Part model, mm, in its own coordinate system. A direction names the side the tool comes from. Give positions to 0.01 mm unless a question says otherwise; leave off trailing zeros. Loops run counter-clockwise (first coordinate to the right, second up) from the corner with the lowest first, then second, coordinate; pieces in that order, holes last. Notation, with made-up numbers: M 59,32 L 103,32 A24 ccw 103,58 Z; hole C 14.25,58 d6. An arc over 180 degrees is marked long. Answer in a Markdown table with one row per item.
from build123d import *

# Parameters (mm, degrees)
BOSS_EXTRUDE1_DEPTH     = 12
SKETCH5_R               = 1
CUT_EXTRUDE1_DEPTH      = 10
CUT_EXTRUDE2_DEPTH      = 3
CUT_EXTRUDE2_DEPTH_BACK = 3
CUT_EXTRUDE3_DEPTH      = 21.976176963
CUT_EXTRUDE3_DEPTH_BACK = 21.976176963
SKETCH7_R               = 1.5
SKETCH10_W              = 7
SKETCH10_H              = 3
CUT_EXTRUDE4_DEPTH      = 3
SKETCH9_R               = 1
CUT_EXTRUDE5_DEPTH      = 27.981475126
SKETCH12_R              = 3
CUT_EXTRUDE6_DEPTH      = 6.5
CUT_EXTRUDE7_DEPTH      = 6.5


with BuildPart() as part:
    # Sketch2 → Boss-Extrude1 (new body)
    with BuildSketch(Plane(origin=(0, 0, 0), x_dir=(1, 0, 0), z_dir=(0, 1, 0))):
        Polygon((0, 10), (11, 10), (11, 0), (-11, 0), (-11, 10), align=None)
    extrude(amount=BOSS_EXTRUDE1_DEPTH)

    # Sketch5 → Cut-Extrude1 (cut)
    with BuildSketch(Plane(origin=(0, 0, -10), x_dir=(-1, 0, 0), z_dir=(0, 0, -1))):
        with Locations((9.5, 1.5)):
            Circle(SKETCH5_R)
    cut_extrude1 = extrude(amount=-CUT_EXTRUDE1_DEPTH, mode=Mode.SUBTRACT)

    # Sketch6 → Cut-Extrude2 (cut, two sides: drawn at the far end of the back side and taken through both)
    with BuildSketch(Plane(origin=(0, 0, 0), x_dir=(0, 0, -1), z_dir=(1, 0, 0)).offset(-CUT_EXTRUDE2_DEPTH_BACK)):
        with BuildLine():
            Line((6, 9.2), (10, 9.2))
            Line((10, 9.2), (10, 2.8))
            Line((10, 2.8), (6, 2.8))
            ThreePointArc((6, 2.8), (2.8, 6), (6, 9.2))
        make_face()
    extrude(amount=CUT_EXTRUDE2_DEPTH + CUT_EXTRUDE2_DEPTH_BACK, mode=Mode.SUBTRACT)

    # Sketch7 → Cut-Extrude3 (cut, two sides: drawn at the far end of the back side and taken through both)
    with BuildSketch(Plane.ZY.offset(-3).offset(-CUT_EXTRUDE3_DEPTH_BACK)):
        with Locations((-6, 6)):
            Circle(SKETCH7_R)
    extrude(amount=CUT_EXTRUDE3_DEPTH + CUT_EXTRUDE3_DEPTH_BACK, mode=Mode.SUBTRACT)

    # Sketch10 → Cut-Extrude4 (cut)
    with BuildSketch(Plane(origin=(0, 0, 0), x_dir=(1, 0, 0), z_dir=(0, 1, 0))):
        with Locations((-7.5, 1.5)):
            Rectangle(SKETCH10_W, SKETCH10_H)
    cut_extrude4 = extrude(amount=CUT_EXTRUDE4_DEPTH, mode=Mode.SUBTRACT)

    # Sketch9 → Cut-Extrude5 (cut, through all)
    with BuildSketch(Plane.ZY.offset(11)):
        with Locations((-1.5, 1.5)):
            Circle(SKETCH9_R)
    extrude(amount=-CUT_EXTRUDE5_DEPTH, mode=Mode.SUBTRACT)

    # Mirror1: Cut-Extrude1, Cut-Extrude4 across plane
    add(cut_extrude1.mirror(Plane(origin=(0, 0, 0), x_dir=(0, 0, 1), z_dir=(1, 0, 0))), mode=Mode.SUBTRACT)
    add(cut_extrude4.mirror(Plane(origin=(0, 0, 0), x_dir=(0, 0, 1), z_dir=(1, 0, 0))), mode=Mode.SUBTRACT)

    # Sketch12 → Cut-Extrude6 (cut)
    with BuildSketch(Plane(origin=(11, 0, 0), x_dir=(0, 0, -1), z_dir=(1, 0, 0))):
        with Locations((6, 6)):
            Circle(SKETCH12_R)
    extrude(amount=-CUT_EXTRUDE6_DEPTH, mode=Mode.SUBTRACT)

    # Sketch13 → Cut-Extrude7 (cut)
    with BuildSketch(Plane.ZY.offset(11)):
        Polygon((-9, 7.732050808), (-9, 4.267949192), (-6, 2.535898385), (-3, 4.267949192), (-3, 7.732050808), (-6, 9.464101615), align=None)
    extrude(amount=-CUT_EXTRUDE7_DEPTH, mode=Mode.SUBTRACT)


solid = part.part
(1) Which spindle directions (+Z, -Z, +X, -X, +Y, -Y) get a long thin tool onto all of the face, cutting with end or side? Do faces 1 (the face through (-7.8, 3.4, -4.5)), 2 (the face through (-8, 3, -2)), 3 (the face through (8, 1, -3)). Say none if no direction does.
Recorded:
| item | result |
|---|---|
| face 1 | -X |
| face 2 | +Z, -X, -Y |
| face 3 | +Z, +X, -Y |
(2) Saw through at C-C (z = -1.5). Write the cut outline in (x, y).
Recorded:
| item | result |
|---|---|
| outline | M -11,3 L -4,3 L -4,2.5 L 4,2.5 L 4,3 L 11,3 L 11,12 L -11,12 Z; M -4,0 L 4,0 L 4,0.5 L -4,0.5 Z |
(3) Saw through at D-D (x = 9.5). Write the cut outline in (y, z).
Recorded:
| item | result |
|---|---|
| outline | M 0,-10 L 0.5,-10 L 0.5,-3 L 0,-3 Z; M 2.5,-10 L 12,-10 L 12,0 L 3,0 L 3,-3 L 2.5,-3 Z; hole C 6,-6 d6 |
(4) Saw through at B-B (y = 1.5). Write the cut outline in (x, z), plus the area to 3 significant figures.
Recorded:
| item | result |
|---|---|
| outline | M -11,-10 L -10.5,-10 L -10.5,-3 L -11,-3 Z; M -8.5,-10 L 8.5,-10 L 8.5,-3 L 4,-3 L 4,-2.5 L -4,-2.5 L -4,-3 L -8.5,-3 Z; M -4,-0.5 L 4,-0.5 L 4,0 L -4,0 Z; M 10.5,-10 L 11,-10 L 11,-3 L 10.5,-3 Z |
| area | 134 mm^2 |
(5) Pull direction X, two halves, no side cores. Call faces 4 (the face through (7.796, 3.338, -7.384)), 5 (the face through (-11, 5.9, -2.7)), 6 (the face through (-8.7, 0.9, -6.5)): +X half, -X half, draft (parallel to the pull), parting line (faces both ways), or undercut.
Recorded:
| item | result |
|---|---|
| face 4 | draft |
| face 5 | -X half |
| face 6 | undercut |
(6) Pin check, flat tips, straight feed: pin 1 Ø0.9 at (x, y) = (8, 1) entering from +Z; pin 2 Ø1.6 at (y, z) = (1.5, -1.5) entering from -X; pin 3 Ø1.5 at (x, z) = (-6, -2) entering from -Y; pin 4 Ø3 at (y, z) = (4.5, -6) entering from -X. Stop position of each tip, or through.
Recorded:
| item | result |
|---|---|
| pin 1 | stops at z = -3 |
| pin 2 | passes through |
| pin 3 | stops at y = 3 |
| pin 4 | stops at x = -4.5 |
(7) Saw through at A-A (x = -9.5). Write the cut outline in (y, z), plus the area to 3 significant figures.
Recorded:
| item | result |
|---|---|
| outline | M 0,-10 L 0.5,-10 L 0.5,-3 L 0,-3 Z; M 2.5,-10 L 12,-10 L 12,0 L 3,0 L 3,-3 L 2.5,-3 Z; hole M 2.54,-6 L 4.27,-9 L 7.73,-9 L 9.46,-6 L 7.73,-3 L 4.27,-3 Z |
| area | 65.8 mm^2 |
(8) Drill centre lines: line 1 along Z through (x, y) = (-3.4, 6); line 2 along Y through (x, z) = (2, -1.5); line 3 along Y through (x, z) = (10.25, -4). Where is each one in solid material? Low to high.
Recorded:
| item | result |
|---|---|
| line 1 | z = -10 to -7.5, -4.5 to 0 |
| line 2 | y = 0 to 0.5, 2.5 to 12 |
| line 3 | y = 0 to 0.84, 2.16 to 3.76, 8.24 to 12 |
